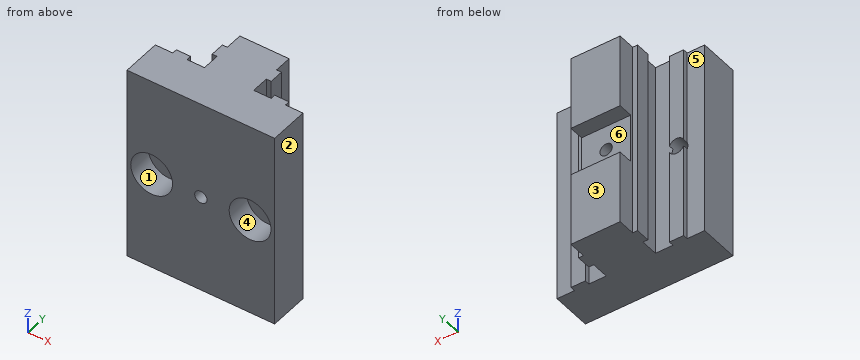
```python
from build123d import *

# Parameters (mm, degrees)
MAIN_DEPTH         = 40
ESQUISSE2_R        = 1.6
TOPHOLE_DEPTH      = 10
ESQUISSE3_R        = 1.25
CENTRALHOLE_DEPTH  = 19
SKETCH1_R          = 4.25
CUT_EXTRUDE1_DEPTH = 5
SKETCH2_W          = 10
SKETCH2_H          = 10
CUT_EXTRUDE2_DEPTH = 3


with BuildPart() as part:
    # Esquisse1 → Main (new body)
    with BuildSketch(Plane.XY):
        Polygon((-15, 0), (-15, 8), (-11.45, 8), (-11.45, 9), (-8.55, 9), (-8.55, 8), (-5, 8), (-5, 11.55), (-6, 11.55), (-6, 14.45), (-5, 14.45), (-5, 18), (0, 18), (0, 0), align=None)
    main = extrude(amount=MAIN_DEPTH)

    # Esquisse2 → TopHole (cut, through all)
    with BuildSketch(Plane(origin=(0, 9, 0), x_dir=(1, 0, 0), z_dir=(0, 1, 0))):
        with Locations((-10, -20)):
            Circle(ESQUISSE2_R)
    tophole = extrude(amount=-TOPHOLE_DEPTH, mode=Mode.SUBTRACT)

    # Symétrie1: Main, TopHole across plane
    add(main.mirror(Plane(origin=(0, 0, 0), x_dir=(0, 0, 1), z_dir=(1, 0, 0))))
    add(tophole.mirror(Plane(origin=(0, 0, 0), x_dir=(0, 0, 1), z_dir=(1, 0, 0))), mode=Mode.SUBTRACT)

    # Esquisse3 → CentralHole (cut, through all)
    with BuildSketch(Plane(origin=(0, 18, 0), x_dir=(1, 0, 0), z_dir=(0, 1, 0))):
        with Locations((0, -20)):
            Circle(ESQUISSE3_R)
    extrude(amount=-CENTRALHOLE_DEPTH, mode=Mode.SUBTRACT)

    # Sketch1 → Cut-Extrude1 (cut)
    with BuildSketch(Plane(origin=(0, 0, 0), x_dir=(-1, 0, 0), z_dir=(0, -1, 0))):
        with Locations((10, -20)):
            Circle(SKETCH1_R)
        with Locations((-10, -20)):
            Circle(SKETCH1_R)
    extrude(amount=-CUT_EXTRUDE1_DEPTH, mode=Mode.SUBTRACT)

    # Sketch2 → Cut-Extrude2 (cut)
    with BuildSketch(Plane(origin=(0, 18, 0), x_dir=(1, 0, 0), z_dir=(0, 1, 0))):
        with Locations((0, -20)):
            Rectangle(SKETCH2_W, SKETCH2_H)
    extrude(amount=-CUT_EXTRUDE2_DEPTH, mode=Mode.SUBTRACT)


solid = part.part
```
Work out the finished part from the listing and answer in its coordinate system (mm). Face numbers are marked on the shaded views. A direction names the side the tool comes from. Give positions to 0.01 mm unless a question says otherwise; leave off trailing zeros. Write each loop counter-clockwise with the first axis right and the second up, starting at its lowest first coordinate (ties: lowest second). Pieces come first, ordered by that corner, then holes. Notation, with made-up numbers: (42, 1) -> (79, 1) arc R15 ccw to (79, 29) -> close; hole circle Ø10 at (84, 32.5). An arc over 180 degrees is marked (long way). Write item = value, one per line.
Q1. For a pull along X with two mould halves and no side action, classify the marked faces 1, 2 and 3 as pulls with the +X half, pulls with the -X half, needs draft (parallel to the pull), parting line crosses it, or undercut.
Computed values:
face_1 = undercut
face_2 = pulls with the +X half
face_3 = needs draft
Q2. Section A-A on x = 10 is taken. Determine the outline of the cut face in (y, z).
Computed values:
outline = (0, 0) -> (9, 0) -> (9, 18.4) -> (5, 18.4) -> (5, 15.75) -> (0, 15.75) -> close; (0, 24.25) -> (5, 24.25) -> (5, 21.6) -> (9, 21.6) -> (9, 40) -> (0, 40) -> close
Q3. Consider line 1 along X through (y, z) = (8.5, 34.5); line 2 along X through (y, z) = (1.05, 20); line 3 along Y through (x, z) = (-5.25, 10). Determine where each line is inside the solid, lowest interval first.
Computed values:
line_1 = -11.45 to -8.55, -5 to 5, 8.55 to 11.45
line_2 = -15 to -14.25, -5.75 to -1.25, 1.25 to 5.75, 14.25 to 15
line_3 = 0 to 8, 11.55 to 14.45
Q4. Section B-B on y = 1.5 is taken. Determine the outline of the cut face in (x, z).
Computed values:
outline = (-15, 0) -> (15, 0) -> (15, 40) -> (-15, 40) -> close; hole circle Ø8.5 at (-10, 20); hole circle Ø2.5 at (0, 20); hole circle Ø8.5 at (10, 20)
Q5. A tool of negligible diameter and unlimited length cuts with its end or side. For the marked faces 4, 5 and 6, from which of +Z, -Z, +X, -X, +Y, -Y can it reach the whole face along a straight path? Write none if from no direction.
Computed values:
face_4 = -Y
face_5 = +Z, -Z, -X, +Y
face_6 = +X, -X, +Y
Q6. Section D-D on x = 0 is taken. Determine the outline of the cut face in (y, z), and give its area (4 significant figures).
Computed values:
outline = (0, 0) -> (18, 0) -> (18, 15) -> (15, 15) -> (15, 18.75) -> (0, 18.75) -> close; (0, 21.25) -> (15, 21.25) -> (15, 25) -> (18, 25) -> (18, 40) -> (0, 40) -> close
area = 652.5 mm^2
Q7. Section C-C on z = 6.5 is taken. Determine the outline of the cut face in (x, y), and give its area (3 significant figures).
Computed values:
outline = (-15, 0) -> (15, 0) -> (15, 8) -> (11.45, 8) -> (11.45, 9) -> (8.55, 9) -> (8.55, 8) -> (5, 8) -> (5, 11.55) -> (6, 11.55) -> (6, 14.45) -> (5, 14.45) -> (5, 18) -> (-5, 18) -> (-5, 14.45) -> (-6, 14.45) -> (-6, 11.55) -> (-5, 11.55) -> (-5, 8) -> (-8.55, 8) -> (-8.55, 9) -> (-11.45, 9) -> (-11.45, 8) -> (-15, 8) -> close
area = 352 mm^2
Q8. Flat-ended cylindrical pins translate along their axes: pin 1 Ø1.5 at (x, z) = (9.5, 12) entering from +Y; pin 2 Ø1 at (y, z) = (15, 8.5) entering from +X; pin 3 Ø0.8 at (y, z) = (8.5, 30.5) entering from -X. Find the tip coordinate at first contact, or state that the pin passes through.
Computed values:
pin_1 = 9
pin_2 = 5
pin_3 = -11.45
